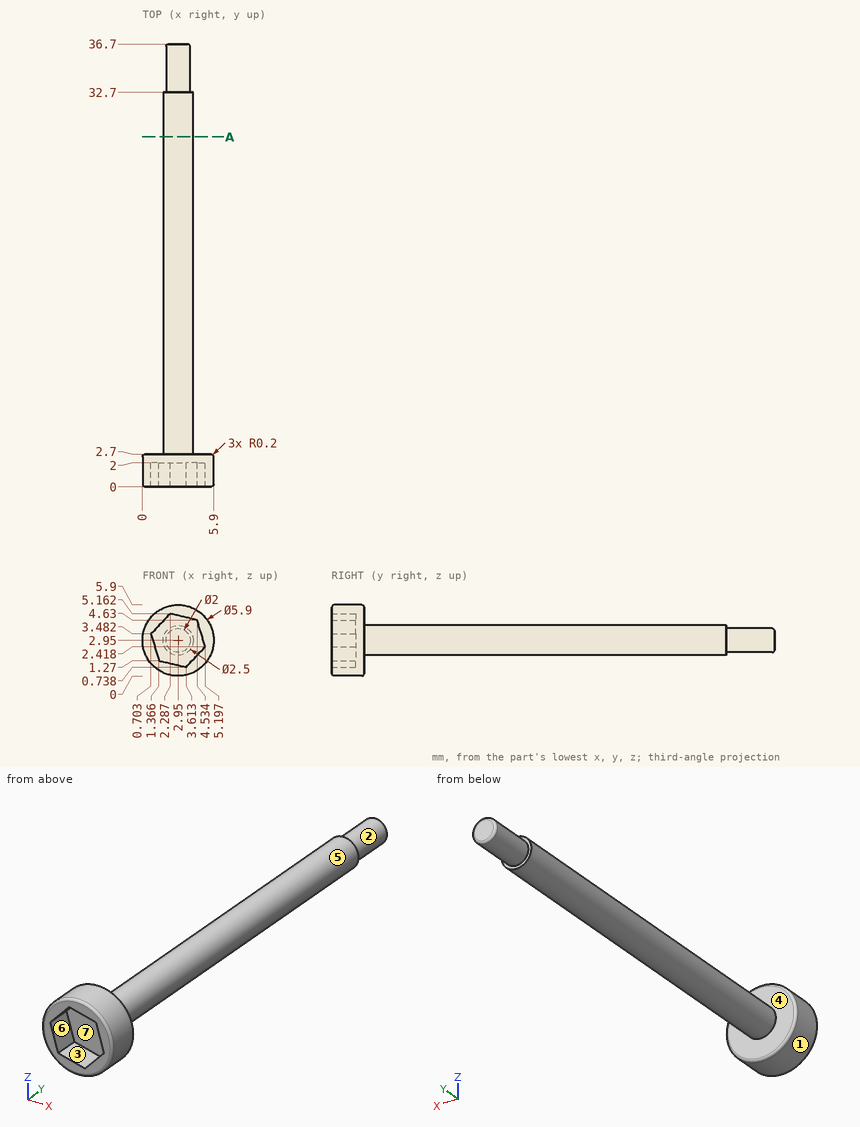
Answer from the drawing. Dimensions are ordinates in mm from the lowest x, y and z of the part. A direction names the side the tool comes from. Coordinates: 2 decimals unless noted, no trailing zeros. Loops run counter-clockwise (first coordinate to the right, second up) from the corner with the lowest first, then second, coordinate; pieces in that order, holes last. Notation, with made-up numbers: (-26, 31.5) - (28, 31.5) arc R3 cw to (28, 35.5) - close; hole circle Ø10 at (88, 7). An arc over 180 degrees is marked (long way). Use a Markdown table: item, result.
Item 1: Find section A-A, the plane y = 29. Determine the outline of the cut face in (x, z).
Evaluation:
| item | result |
|---|---|
| outline | circle Ø2.5 at (2.95, 2.95) |
Item 2: Given pin 1 Ø2 at (y, z) = (31, 2.5) entering from -X; pin 2 Ø3 at (y, z) = (11, 4.5) entering from +X; pin 3 Ø3 at (y, z) = (15.5, 0.5) entering from +X; pin 4 Ø3.5 at (x, z) = (2.5, 3) entering from -Y, each flat-ended and moving along its own axis, determine where each tip first touches the part or whether it passes through.
Evaluation:
| item | result |
|---|---|
| pin 1 | stops at x = 1.7 |
| pin 2 | stops at x = 4.2 |
| pin 3 | stops at x = 3.76 |
| pin 4 | stops at y = 0 |
Item 3: The mould has two halves that part along Z. Classify the marked faces 4, 5, 6 and 7: +Z half, -Z half, draft (parallel to the pull), parting line (faces both ways), or undercut.
Evaluation:
| item | result |
|---|---|
| face 4 | draft |
| face 5 | parting line |
| face 6 | undercut |
| face 7 | undercut |
Item 4: For the marked faces 1, 2 and 3, determine the directions among +Z, -Z, +X, -X, +Y, -Y from which every point of the face is accessible in a straight line to the end or side of a thin tool.
Evaluation:
| item | result |
|---|---|
| face 1 | +Y, -Y |
| face 2 | +Y |
| face 3 | -Y |
Item 5: Consider probe 1 along Y at (x, z) = (2.7, 0.35); probe 2 along Y at (x, z) = (2.5, 4); probe 3 along Z at (x, y) = (2.9, 4). Determine where each line is inside the solid, lowest interval first. Write a range as from..to.
Evaluation:
| item | result |
|---|---|
| probe 1 | y = 0..2.7 |
| probe 2 | y = 2..32.7 |
| probe 3 | z = 1.7..4.2 |
